from build123d import *

# Parameters (mm, degrees)
SKETCH1_W           = 135
SKETCH1_H           = 70
BOSS_EXTRUDE1_DEPTH = 15
FILLET2_R           = 10
FILLET3_R           = 10
FILLET4_R           = 10
FILLET5_R           = 10
FILLET12_R          = 10
FILLET13_R          = 10


with BuildPart() as part:
    # Sketch1 → Boss-Extrude1 (new body)
    with BuildSketch(Plane.XY):
        with Locations((18.404407689, 12.303703611)):
            Rectangle(SKETCH1_W, SKETCH1_H)
    extrude(amount=BOSS_EXTRUDE1_DEPTH)

    # Fillet2
    fillet2_edges = [part.edges().sort_by_distance(p)[0] for p in [
        (-49.095592311, -22.696296389, 7.5),
    ]]
    fillet(fillet2_edges, radius=FILLET2_R)

    # Fillet3
    fillet3_edges = [part.edges().sort_by_distance(p)[0] for p in [
        (-49.095592311, 47.303703611, 7.5),
    ]]
    fillet(fillet3_edges, radius=FILLET3_R)

    # Fillet4
    fillet4_edges = [part.edges().sort_by_distance(p)[0] for p in [
        (85.904407689, 47.303703611, 7.5),
    ]]
    fillet(fillet4_edges, radius=FILLET4_R)

    # Fillet5
    fillet5_edges = [part.edges().sort_by_distance(p)[0] for p in [
        (85.904407689, -22.696296389, 7.5),
    ]]
    fillet(fillet5_edges, radius=FILLET5_R)

    # Fillet12
    fillet12_edges = [part.edges().sort_by_distance(p)[0] for p in [
        (18.404407689, -22.696296389, 0),
        (-46.166660123, -19.7673642, 0),
        (-49.095592311, 12.303703611, 0),
        (-46.166660123, 44.374771423, 0),
        (18.404407689, 47.303703611, 0),
        (82.975475501, 44.374771423, 0),
        (85.904407689, 12.303703611, 0),
        (82.975475501, -19.7673642, 0),
    ]]
    fillet(fillet12_edges, radius=FILLET12_R)

    # Fillet13
    # the kernel refuses this fillet: 10 mm, written as the material it takes off along each edge
    with BuildSketch(Plane(origin=(75.904407689, 37.303703611, 15), x_dir=(0, 1, 0), z_dir=(-1, 0, 0))) as fillet13_piece_1:
        with BuildLine():
            CenterArc((1.339745962, 10), FILLET13_R, 270, 60)
            Line((10, 5), (10.173205081, 4.9))
            ThreePointArc((10.173205081, 4.9), (10.2, 2.5), (10.2, 0))
            Line((10.2, 0), (10, -0.2))
            Line((10, -0.2), (1.339745962, -0.2))
            Line((1.339745962, -0.2), (1.339745962, 0))
        make_face()
    revolve(axis=Axis((75.904407689, 37.303703611, 15), (0, 0, -1)), revolution_arc=90, mode=Mode.SUBTRACT)
    with BuildSketch(Plane(origin=(75.904407689, -12.696296389, 15), x_dir=(1, 0, 0), z_dir=(0, 1, 0))) as fillet13_piece_2:
        with BuildLine():
            CenterArc((1.339745962, 10), FILLET13_R, 270, 60)
            Line((1.339745962, 0), (1.339745962, -0.2))
            Line((1.339745962, -0.2), (10, -0.2))
            Line((10, -0.2), (10.2, 0))
            ThreePointArc((10.2, 0), (10.2, 2.5), (10.173205081, 4.9))
            Line((10.173205081, 4.9), (10, 5))
        make_face()
    revolve(axis=Axis((75.904407689, -12.696296389, 15), (0, 0, -1)), revolution_arc=90, mode=Mode.SUBTRACT)
    with BuildSketch(Plane(origin=(-39.095592311, -12.696296389, 15), x_dir=(0, -1, 0), z_dir=(1, 0, 0))) as fillet13_piece_3:
        with BuildLine():
            CenterArc((1.339745962, 10), FILLET13_R, 270, 60)
            Line((10, 5), (10.173205081, 4.9))
            ThreePointArc((10.173205081, 4.9), (10.2, 2.5), (10.2, 0))
            Line((10.2, 0), (10, -0.2))
            Line((10, -0.2), (1.339745962, -0.2))
            Line((1.339745962, -0.2), (1.339745962, 0))
        make_face()
    revolve(axis=Axis((-39.095592311, -12.696296389, 15), (0, 0, -1)), revolution_arc=90, mode=Mode.SUBTRACT)
    with BuildSketch(Plane(origin=(-39.095592311, 37.303703611, 15), x_dir=(-1, 0, 0), z_dir=(0, -1, 0))) as fillet13_piece_4:
        with BuildLine():
            CenterArc((1.339745962, 10), FILLET13_R, 270, 60)
            Line((10, 5), (10.173205081, 4.9))
            ThreePointArc((10.173205081, 4.9), (10.2, 2.5), (10.2, 0))
            Line((10.2, 0), (10, -0.2))
            Line((10, -0.2), (1.339745962, -0.2))
            Line((1.339745962, -0.2), (1.339745962, 0))
        make_face()
    revolve(axis=Axis((-39.095592311, 37.303703611, 15), (0, 0, -1)), revolution_arc=90, mode=Mode.SUBTRACT)
    with BuildSketch(Plane(origin=(-49.095592311, -12.696296389, 15), x_dir=(0, 0, -1), z_dir=(0, 1, 0)), Plane(origin=(85.904407689, 37.303703611, 15), x_dir=(0, 0, -1), z_dir=(0, -1, 0))) as fillet13_piece_5:
        with BuildLine():
            CenterArc((10, -8.660254038), FILLET13_R, 120, 60)
            Line((0, -8.660254038), (-0.2, -8.660254038))
            Line((-0.2, -8.660254038), (-0.2, 0))
            Line((-0.2, 0), (0, 0.2))
            ThreePointArc((0, 0.2), (2.5, 0.2), (4.9, 0.173205081))
            Line((4.9, 0.173205081), (5, 0))
        make_face()
    extrude(amount=50, mode=Mode.SUBTRACT)
    with BuildSketch(Plane(origin=(75.904407689, -22.696296389, 15), x_dir=(0, 0, -1), z_dir=(-1, 0, 0)), Plane(origin=(-39.095592311, 47.303703611, 15), x_dir=(0, 0, -1), z_dir=(1, 0, 0))) as fillet13_piece_6:
        with BuildLine():
            CenterArc((10, -8.660254038), FILLET13_R, 120, 60)
            Line((0, -8.660254038), (-0.2, -8.660254038))
            Line((-0.2, -8.660254038), (-0.2, 0))
            Line((-0.2, 0), (0, 0.2))
            ThreePointArc((0, 0.2), (2.5, 0.2), (4.9, 0.173205081))
            Line((4.9, 0.173205081), (5, 0))
        make_face()
    extrude(amount=115, mode=Mode.SUBTRACT)


solid = part.part
Design review of the part built by this model. Coordinates are the model's own, in mm. Give positions to 0.01 mm unless a question says otherwise; leave off trailing zeros. Loops run counter-clockwise (first coordinate to the right, second up) from the corner with the lowest first, then second, coordinate; pieces in that order, holes last. Notation, with made-up numbers: M 54,43.25 L 113,43.25 A16 cw 113,54.25 Z; hole C 0,29.25 d6. An arc over 180 degrees is marked long. Write item = value, one per line.
Q1. Insertion check: pin 1 (8 mm diameter, centred on x = 7, z = 12.5, fed in from +Y); pin 2 (1.5 mm diameter, centred on y = 14.5, z = 8, fed in from +X); pin 3 (3 mm diameter, centred on x = 51, z = 6.5, fed in from +Y); pin 4 (3 mm diameter, centred on x = 50, z = 12.5, fed in from -Y). Each pin has a flat end and moves straight along its axis. Give the tip position at first contact, or say it passes through.
Output values:
pin_1 = 47.3
pin_2 = 85.83
pin_3 = 47.1
pin_4 = -22.04
Q2. To check wall thickness, follow line 1 (Y direction, x = 37, z = 9.75); line 2 (X direction, y = 7, z = 5.5); line 3 (Y direction, x = 14, z = 14). State the ranges of each line that lie inside material, in increasing order. Write a range as [from, to].
Output values:
line_1 = [-22.69, 47.3]
line_2 = [-48.03, 84.83]
line_3 = [-18.39, 43]
Q3. We need section A-A (y = 15). Give the boundary of the cut face in (x, z), plus the area to 3 significant figures.
Output values:
outline = M -49.1,10 A10 ccw -39.1,0 L 75.9,0 A10 ccw 85.9,10 A10 ccw 77.24,15 L -40.44,15 A10 ccw Z
area = 1,960 mm^2
Q4. We need section B-B (z = 5). Give the boundary of the cut face in (x, y), plus the area to 3 significant figures.
Output values:
outline = M -47.76,-12.7 A8.66 ccw -39.1,-21.36 L 75.9,-21.36 A8.66 ccw 84.56,-12.7 L 84.56,37.3 A8.66 ccw 75.9,45.96 L -39.1,45.96 A8.66 ccw -47.76,37.3 Z
area = 8,840 mm^2
Q5. We need section C-C (x = 13.5). Give the boundary of the cut face in (y, z).
Output values:
outline = M -22.7,10 A10 ccw -12.7,0 L 37.3,0 A10 ccw 47.3,10 A10 ccw 38.64,15 L -14.04,15 A10 ccw Z
